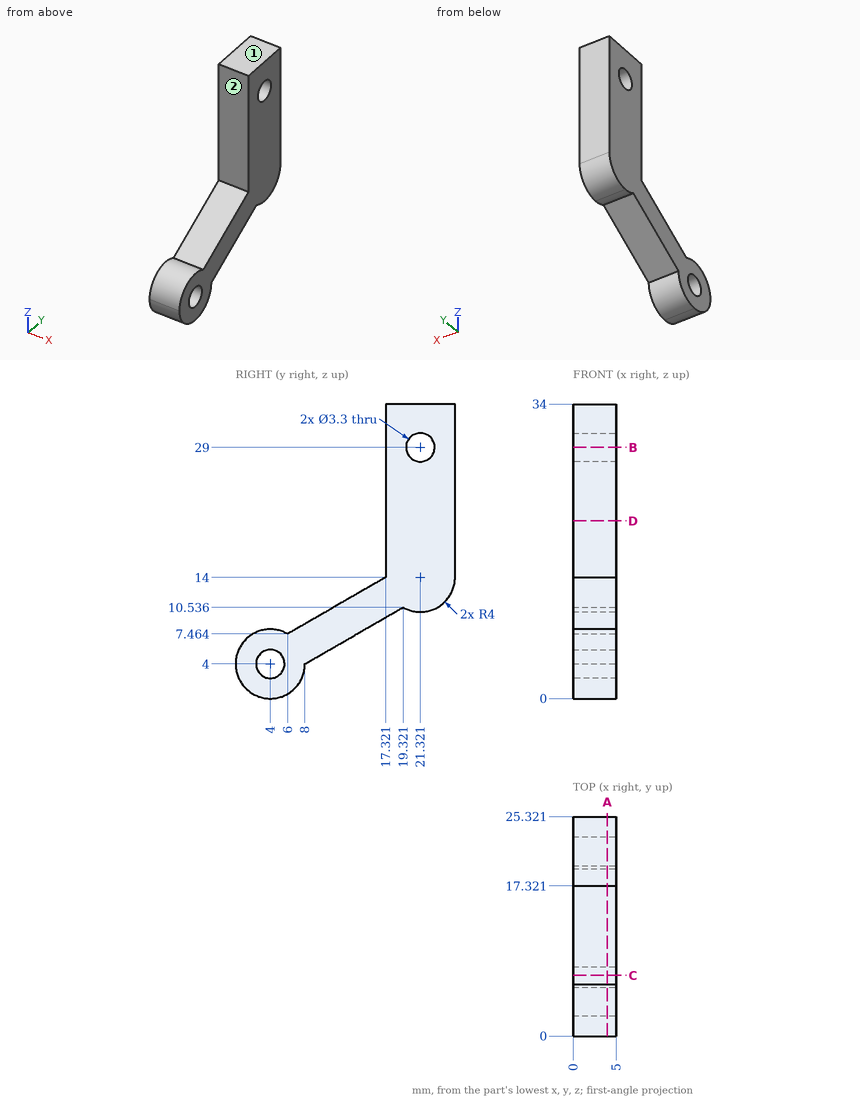
Print and shaded views of the part. All mm, measured from the part's lowest x, y and z. A direction names the side the tool comes from. Give positions to 0.01 mm unless a question says otherwise; leave off trailing zeros. Loops run counter-clockwise (first coordinate to the right, second up) from the corner with the lowest first, then second, coordinate; pieces in that order, holes last. Notation, with made-up numbers: (62, 82) - (103, 82) arc R18 ccw to (103, 108) - close; hole circle Ø8 at (56, -10). An arc over 180 degrees is marked (long way). Use a Markdown table: item, result.
(1) Band-saw the part on D-D (z = 20.5). Give the cut face in (x, y), and give its area (3 significant figures).
Taken from the geometry:
| item | result |
|---|---|
| outline | (0, 17.32) - (5, 17.32) - (5, 25.32) - (0, 25.32) - close |
| area | 40.0 mm2 |
(2) Band-saw the part on A-A (x = 3.95). Give the number of separate pieces and of enclosed holes in the cut face, and give its area (3 significant figures).
Taken from the geometry:
| item | result |
|---|---|
| separate pieces | 1 |
| enclosed holes | 2 |
| area | 268 mm2 |
(3) Which spindle directions (+Z, -Z, +X, -X, +Y, -Y) get a long thin tool onto all of the face, cutting with end or side? Do the marked faces 1 and 2. Say none if no direction does.
Taken from the geometry:
| item | result |
|---|---|
| face 1 | +Z, +X, -X, +Y, -Y |
| face 2 | +Z, +X, -X, -Y |
(4) Wall check: line 1 along Y through (x, z) = (4.65, 29); line 2 along Z through (x, y) = (2.1, 3) (1 decimal); line 3 along Z through (x, y) = (3.95, 3.5). Give the ranges that are in metal, low to high.
Taken from the geometry:
| item | result |
|---|---|
| line 1 | 17.32 to 19.67, 22.97 to 25.32 |
| line 2 | 0.1 to 2.7, 5.3 to 7.9 |
| line 3 | 0.03 to 2.43, 5.57 to 7.97 |
(5) Drop a flat-ended pin along its axis: pin 1 Ø1.5 at (x, y) = (3.5, 10) entering from -Z. Give the stop position or say it passes through.
Taken from the geometry:
| item | result |
|---|---|
| pin 1 | z = 4.72 |
(6) Band-saw the part on C-C (y = 7). Give the cut face in (x, z) (1 decimal).
Taken from the geometry:
| item | result |
|---|---|
| outline | (0, 1.4) - (5, 1.4) - (5, 8) - (0, 8) - close |
(7) Band-saw the part on B-B (z = 29). Give the cut face in (x, y), and give its area (3 significant figures).
Taken from the geometry:
| item | result |
|---|---|
| outline | (0, 17.32) - (5, 17.32) - (5, 19.67) - (0, 19.67) - close; (0, 22.97) - (5, 22.97) - (5, 25.32) - (0, 25.32) - close |
| area | 23.5 mm2 |
